Part model, mm, in its own coordinate system. Face numbers are marked on the shaded views. Coordinates: 2 decimals unless noted, no trailing zeros. Loops run counter-clockwise (first coordinate to the right, second up) from the corner with the lowest first, then second, coordinate; pieces in that order, holes last. Notation, with made-up numbers: (12.5, 50) - (58.5, 50) arc R13 ccw to (58.5, 70) - close; hole circle Ø7 at (13.5, -30.5). An arc over 180 degrees is marked (long way). Use a Markdown table: item, result. Add a question column.
1. Band-saw the part on B-B, the plane z = 1.2. Count the separate pieces of the cut face and the enclosed holes in it, plus the area to 3 significant figures.
2. Drop flat-ended pins along their axis: pin 1 (1.5 mm diameter, centred on x = 91.5, z = 2, fed in from +Y); pin 2 (1 mm diameter, centred on x = -49.5, z = 1, fed in from -Y). Give the stop position or say it passes through.
3. Pull direction Z, two halves, no side cores. Call the marked faces 1 and 2: pulls with the +Z half, pulls with the -Z half, needs draft (parallel to the pull), parting line crosses it, or undercut.
4. Wall check: probe 1 along Y at (x, z) = (98.5, 1.1) (3 decimals); probe 2 along Y at (x, z) = (-150.5, 2.95); probe 3 along X at (y, z) = (-184, 1.85). Give the ranges that are in metal, low to high. Write a range as [from, to].
5. Band-saw the part on A-A, the plane x = 45. Give the cut face in (y, z) (3 decimals), plus the area to 3 significant figures.
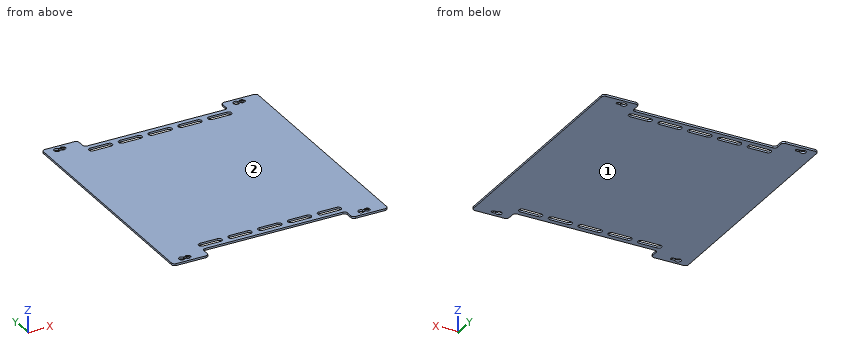
from build123d import *

# Parameters (mm, degrees)
BOSS_EXTRUDE1_DEPTH = 3.175
SKETCH2_R           = 4.8
CUT_EXTRUDE1_DEPTH  = 1
CUT_EXTRUDE2_DEPTH  = 3.175


with BuildPart() as part:
    # Model → Boss-Extrude1 (new body)
    with BuildSketch(Plane.XY):
        with BuildLine():
            Line((175.500000042, 200.504864864), (125.500000042, 200.504864864))
            ThreePointArc((125.500000042, 200.504864864), (121.964466136, 199.04039877), (120.500000042, 195.504864864))
            Line((120.500000042, 195.504864864), (120.500000042, 185.00000269))
            ThreePointArc((120.500000042, 185.00000269), (119.035533948, 181.464468784), (115.500000042, 180.00000269))
            Line((115.500000042, 180.00000269), (-115.500000042, 180.00000269))
            ThreePointArc((-115.500000042, 180.00000269), (-119.035533948, 181.464468784), (-120.500000042, 185.00000269))
            Line((-120.500000042, 185.00000269), (-120.500000042, 195.504864864))
            ThreePointArc((-120.500000042, 195.504864864), (-121.964466136, 199.04039877), (-125.500000042, 200.504864864))
            Line((-125.500000042, 200.504864864), (-175.500000042, 200.504864864))
            ThreePointArc((-175.500000042, 200.504864864), (-179.035533948, 199.04039877), (-180.500000042, 195.504864864))
            Line((-180.500000042, 195.504864864), (-180.500000042, -195.504859484))
            ThreePointArc((-180.500000042, -195.504859484), (-179.035533948, -199.04039339), (-175.500000042, -200.504859484))
            Line((-175.500000042, -200.504859484), (-125.500000042, -200.504859484))
            ThreePointArc((-125.500000042, -200.504859484), (-121.964466136, -199.04039339), (-120.500000042, -195.504859484))
            Line((-120.500000042, -195.504859484), (-120.500000042, -184.99999731))
            ThreePointArc((-120.500000042, -184.99999731), (-119.035533948, -181.464463404), (-115.500000042, -179.99999731))
            Line((-115.500000042, -179.99999731), (115.500000042, -179.99999731))
            ThreePointArc((115.500000042, -179.99999731), (119.035533948, -181.464463404), (120.500000042, -184.99999731))
            Line((120.500000042, -184.99999731), (120.500000042, -195.504864864))
            ThreePointArc((120.500000042, -195.504864864), (121.964466136, -199.04039877), (125.500000042, -200.504864864))
            Line((125.500000042, -200.504864864), (175.500000042, -200.504864864))
            ThreePointArc((175.500000042, -200.504864864), (179.035533948, -199.04039877), (180.500000042, -195.504864864))
            Line((180.500000042, -195.504864864), (180.500000042, 195.504864864))
            ThreePointArc((180.500000042, 195.504864864), (179.035533948, 199.04039877), (175.500000042, 200.504864864))
        make_face()
        with BuildLine():
            Line((144.600753463, 187.915208316), (150.5, 187.915208316))
            ThreePointArc((150.5, 187.915208316), (153.089656548, 190.504864864), (150.5, 193.094521412))
            Line((150.5, 193.094521412), (144.600753463, 193.094521412))
            ThreePointArc((144.600753463, 193.094521412), (135.65, 190.504864864), (144.600753463, 187.915208316))
        make_face(mode=Mode.SUBTRACT)
        with BuildLine():
            Line((150.5, -187.905478588), (144.600753463, -187.905478588))
            ThreePointArc((144.600753463, -187.905478588), (135.65, -190.495135136), (144.600753463, -193.084791684))
            Line((144.600753463, -193.084791684), (150.5, -193.084791684))
            ThreePointArc((150.5, -193.084791684), (153.089656548, -190.495135136), (150.5, -187.905478588))
        make_face(mode=Mode.SUBTRACT)
        with BuildLine():
            Line((-150.5, -187.905478588), (-156.399246537, -187.905478588))
            ThreePointArc((-156.399246537, -187.905478588), (-165.35, -190.495135136), (-156.399246537, -193.084791684))
            Line((-156.399246537, -193.084791684), (-150.5, -193.084791684))
            ThreePointArc((-150.5, -193.084791684), (-147.910343452, -190.495135136), (-150.5, -187.905478588))
        make_face(mode=Mode.SUBTRACT)
        with BuildLine():
            Line((-150.5, 193.094521412), (-156.399246537, 193.094521412))
            ThreePointArc((-156.399246537, 193.094521412), (-165.35, 190.504864864), (-156.399246537, 187.915208316))
            Line((-156.399246537, 187.915208316), (-150.5, 187.915208316))
            ThreePointArc((-150.5, 187.915208316), (-147.910343452, 190.504864864), (-150.5, 193.094521412))
        make_face(mode=Mode.SUBTRACT)
    extrude(amount=BOSS_EXTRUDE1_DEPTH)

    # Sketch2 → Cut-Extrude1 (cut)
    with BuildSketch(Plane.XY.offset(3.175)):
        with Locations((-150.5, 190.504864864)):
            Circle(SKETCH2_R)
        with Locations((150.5, 190.504864864)):
            Circle(SKETCH2_R)
        with Locations((150.5, -190.495135136)):
            Circle(SKETCH2_R)
        with Locations((-150.5, -190.495135136)):
            Circle(SKETCH2_R)
    extrude(amount=-CUT_EXTRUDE1_DEPTH, mode=Mode.SUBTRACT)

    # Sketch3 → Cut-Extrude2 (cut)
    with BuildSketch(Plane.XY.offset(3.175)):
        with BuildLine():
            Line((-15, 162.5), (15, 162.5))
            ThreePointArc((15, 162.5), (19.7625, 167.2625), (15, 172.025))
            Line((15, 172.025), (-15, 172.025))
            ThreePointArc((-15, 172.025), (-19.7625, 167.2625), (-15, 162.5))
        make_face()
        with BuildLine():
            Line((35, 172.025), (65, 172.025))
            ThreePointArc((65, 172.025), (69.7625, 167.2625), (65, 162.5))
            Line((65, 162.5), (35, 162.5))
            ThreePointArc((35, 162.5), (30.2375, 167.2625), (35, 172.025))
        make_face()
        with BuildLine():
            Line((85, 172.025), (115, 172.025))
            ThreePointArc((115, 172.025), (119.7625, 167.2625), (115, 162.5))
            Line((115, 162.5), (85, 162.5))
            ThreePointArc((85, 162.5), (80.2375, 167.2625), (85, 172.025))
        make_face()
        with BuildLine():
            Line((-65, 172.025), (-35, 172.025))
            ThreePointArc((-35, 172.025), (-30.2375, 167.2625), (-35, 162.5))
            Line((-35, 162.5), (-65, 162.5))
            ThreePointArc((-65, 162.5), (-69.7625, 167.2625), (-65, 172.025))
        make_face()
        with BuildLine():
            Line((-115, 172.025), (-85, 172.025))
            ThreePointArc((-85, 172.025), (-80.2375, 167.2625), (-85, 162.5))
            Line((-85, 162.5), (-115, 162.5))
            ThreePointArc((-115, 162.5), (-119.7625, 167.2625), (-115, 172.025))
        make_face()
        with BuildLine():
            Line((-115, -162.5), (-85, -162.5))
            ThreePointArc((-85, -162.5), (-80.2375, -167.2625), (-85, -172.025))
            Line((-85, -172.025), (-115, -172.025))
            ThreePointArc((-115, -172.025), (-119.7625, -167.2625), (-115, -162.5))
        make_face()
        with BuildLine():
            Line((-65, -162.5), (-35, -162.5))
            ThreePointArc((-35, -162.5), (-30.2375, -167.2625), (-35, -172.025))
            Line((-35, -172.025), (-65, -172.025))
            ThreePointArc((-65, -172.025), (-69.7625, -167.2625), (-65, -162.5))
        make_face()
        with BuildLine():
            Line((85, -162.5), (115, -162.5))
            ThreePointArc((115, -162.5), (119.7625, -167.2625), (115, -172.025))
            Line((115, -172.025), (85, -172.025))
            ThreePointArc((85, -172.025), (80.2375, -167.2625), (85, -162.5))
        make_face()
        with BuildLine():
            Line((35, -162.5), (65, -162.5))
            ThreePointArc((65, -162.5), (69.7625, -167.2625), (65, -172.025))
            Line((65, -172.025), (35, -172.025))
            ThreePointArc((35, -172.025), (30.2375, -167.2625), (35, -162.5))
        make_face()
        with BuildLine():
            Line((-15, -172.025), (15, -172.025))
            ThreePointArc((15, -172.025), (19.7625, -167.2625), (15, -162.5))
            Line((15, -162.5), (-15, -162.5))
            ThreePointArc((-15, -162.5), (-19.7625, -167.2625), (-15, -172.025))
        make_face()
    extrude(amount=-CUT_EXTRUDE2_DEPTH, mode=Mode.SUBTRACT)


solid = part.part
Geometry check:
| question | item | result |
|---|---|---|
| 1 | separate pieces | 1 |
| 1 | enclosed holes | 14 |
| 1 | area | 131,000 mm^2 |
| 2 | pin 1 | stops at y = 180 |
| 2 | pin 2 | stops at y = -180 |
| 3 | face 1 | pulls with the -Z half |
| 3 | face 2 | pulls with the +Z half |
| 4 | probe 1 | y = [-180, -172.025], [-162.5, 162.5], [172.025, 180] |
| 4 | probe 2 | y = [-200.5, -195.3], [-185.7, 185.7], [195.3, 200.5] |
| 4 | probe 3 | x = [-180.5, -120.4], [120.4, 180.5] |
| 5 | outline | (-180, 0) - (-172.025, 0) - (-172.025, 3.175) - (-180, 3.175) - close; (-162.5, 0) - (162.5, 0) - (162.5, 3.175) - (-162.5, 3.175) - close; (172.025, 0) - (180, 0) - (180, 3.175) - (172.025, 3.175) - close |
| 5 | area | 1,080 mm^2 |
